Check sheet for the drawn part. Datum: minimum x, y, z corner. Units: mm. A direction names the side the tool comes from. Coordinates: 2 decimals unless noted, no trailing zeros. Loops run counter-clockwise (first coordinate to the right, second up) from the corner with the lowest first, then second, coordinate; pieces in that order, holes last.
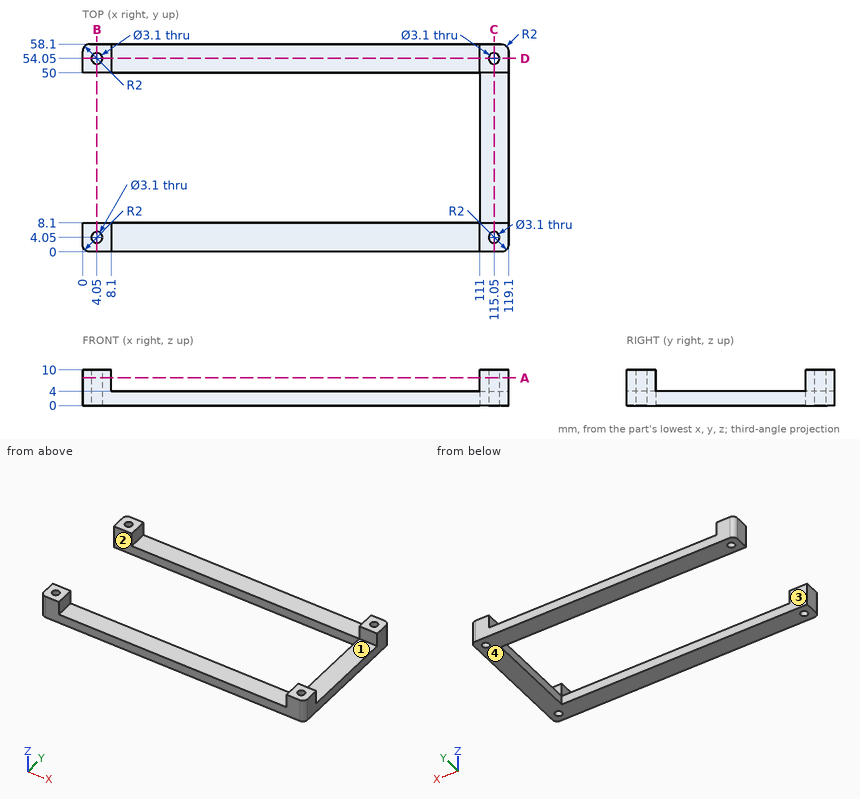
(1) Scan lines: L1, parallel to Y at x = 115.05, z = 7.75; L2, parallel to Y at x = 115.05, z = 2; L3, parallel to Y at x = 64.5, z = 2.75. Record each from-to range of solid material in increasing order.
Findings:
L1: y = 0 to 2.5, 5.6 to 8.1, 50 to 52.5, 55.6 to 58.1
L2: y = 0 to 2.5, 5.6 to 52.5, 55.6 to 58.1
L3: y = 0 to 8.1, 50 to 58.1
(2) Access from +Z, -Z, +X, -X, +Y, -Y to the whole of each face (thin tool, end or side, straight path). Record for the marked faces 1 and 2.
Findings:
face 1: +Z, +X, -X
face 2: +Z, -Z, -X
(3) Draft check along Y on the marked faces 3 and 4. Enter one of: +Y half, -Y half, draft (parallel to the pull), parting line (faces both ways), or undercut.
Findings:
face 3: undercut
face 4: draft
(4) Gauge pin test, flat ends, axial feed: pin 1 Ø1.5 at (x, z) = (44, 4.5) entering from +Y; pin 2 Ø5 at (x, y) = (49, 46.5) entering from +Z; pin 3 Ø6.5 at (x, y) = (115.5, 31.5) entering from +Z; pin 4 Ø2 at (y, z) = (30.5, 2.5) entering from -X. Record the tip position at first contact, or that the pin passes through.
Findings:
pin 1: stops at y = 58.1
pin 2: passes through
pin 3: stops at z = 4
pin 4: stops at x = 111
(5) Sectioned sample at B-B on x = 4.05. Record the cut outline in (y, z), and give its area (3 significant figures).
Findings:
outline: (0, 0) - (2.5, 0) - (2.5, 10) - (0, 10) - close; (5.6, 0) - (8.1, 0) - (8.1, 10) - (5.6, 10) - close; (50, 0) - (52.5, 0) - (52.5, 10) - (50, 10) - close; (55.6, 0) - (58.1, 0) - (58.1, 10) - (55.6, 10) - close
area: 100 mm2
(6) Sectioned sample at C-C on x = 115.05. Record the cut outline in (y, z).
Findings:
outline: (0, 0) - (2.5, 0) - (2.5, 10) - (0, 10) - close; (5.6, 0) - (52.5, 0) - (52.5, 10) - (50, 10) - (50, 4) - (8.1, 4) - (8.1, 10) - (5.6, 10) - close; (55.6, 0) - (58.1, 0) - (58.1, 10) - (55.6, 10) - close
(7) Sectioned sample at D-D on y = 54.05. Record the cut outline in (x, z), and give its area (3 significant figures).
Findings:
outline: (0, 0) - (2.5, 0) - (2.5, 10) - (0, 10) - close; (5.6, 0) - (113.5, 0) - (113.5, 10) - (111, 10) - (111, 4) - (8.1, 4) - (8.1, 10) - (5.6, 10) - close; (116.6, 0) - (119.1, 0) - (119.1, 10) - (116.6, 10) - close
area: 512 mm2
(8) Sectioned sample at A-A on z = 7.75. Record the cut outline in (x, y), and give its area (3 significant figures).
Findings:
outline: (0, 2) arc R2 ccw to (2, 0) - (8.1, 0) - (8.1, 8.1) - (0, 8.1) - close; (0, 50) - (8.1, 50) - (8.1, 58.1) - (2, 58.1) arc R2 ccw to (0, 56.1) - close; (111, 0) - (117.1, 0) arc R2 ccw to (119.1, 2) - (119.1, 8.1) - (111, 8.1) - close; (111, 50) - (119.1, 50) - (119.1, 56.1) arc R2 ccw to (117.1, 58.1) - (111, 58.1) - close; hole circle Ø3.1 at (4.05, 4.05); hole circle Ø3.1 at (4.05, 54.05); hole circle Ø3.1 at (115.05, 4.05); hole circle Ø3.1 at (115.05, 54.05)
area: 229 mm2
